```python
from build123d import *

# Parameters (mm, degrees)
F0_R     = 34.925
F0_R_2   = 16.002
F1_DEPTH = 28.829
F2_DEPTH = 7.112
F0_R_3   = 112.649
F3_DEPTH = 7.493


with BuildPart() as f1:
    # F0 (on Top) → F1 (new body, symmetric)
    with BuildSketch(Plane.XY):
        Circle(F0_R)
        Circle(F0_R_2, mode=Mode.SUBTRACT)
    extrude(amount=F1_DEPTH, both=True)

    # F0 (on Top) → F2 (join, symmetric)
    with BuildSketch(Plane.XY):
        with BuildLine():
            ThreePointArc((41.091917, -3.883291), (41.229204, -1.943802), (41.275, 0))
            ThreePointArc((41.275, 0), (33.800319, 23.688901), (14.083526, 38.797937))
            ThreePointArc((14.083526, 38.797937), (-1.674687, 41.241012), (-17.18293, 37.52829))
            ThreePointArc((-17.18293, 37.52829), (-36.553107, 19.170184), (-40.641762, -7.202277))
            ThreePointArc((-40.641762, -7.202277), (-34.87842, -22.070827), (-23.908987, -33.644999))
            ThreePointArc((-23.908987, -33.644999), (1.674687, -41.241012), (26.558236, -31.59566))
            ThreePointArc((26.558236, -31.59566), (36.553107, -19.170184), (41.091917, -3.883291))
        make_face()
        Circle(F0_R, mode=Mode.SUBTRACT)
        with BuildLine():
            ThreePointArc((-17.18293, 37.52829), (-1.674687, 41.241012), (14.083526, 38.797937))
            Line((14.083526, 38.797937), (14.083526, 96.642205))
            ThreePointArc((14.083526, 96.642205), (-4.052266, 97.578895), (-22.047948, 95.141734))
            Line((-22.047948, 95.141734), (-17.18293, 37.52829))
        make_face()
        with BuildLine():
            ThreePointArc((-23.908987, -33.644999), (-34.87842, -22.070827), (-40.641762, -7.202277))
            Line((-40.641762, -7.202277), (-90.736368, -36.124411))
            ThreePointArc((-90.736368, -36.124411), (-82.479669, -52.298813), (-71.371184, -66.66495))
            Line((-71.371184, -66.66495), (-23.908987, -33.644999))
        make_face()
        with BuildLine():
            Line((93.419133, -28.476784), (41.091917, -3.883291))
            ThreePointArc((41.091917, -3.883291), (36.553107, -19.170184), (26.558236, -31.59566))
            Line((26.558236, -31.59566), (76.652842, -60.517794))
            ThreePointArc((76.652842, -60.517794), (86.531935, -45.280082), (93.419133, -28.476784))
        make_face()
    extrude(amount=F2_DEPTH, both=True)

    # F0 (on Top) → F3 (join, symmetric)
    with BuildSketch(Plane.XY):
        Circle(F0_R_3)
        with BuildLine():
            ThreePointArc((-22.047948, 95.141734), (-4.052266, 97.578895), (14.083526, 96.642205))
            ThreePointArc((14.083526, 96.642205), (73.869821, 63.88514), (97.663, 0))
            ThreePointArc((97.663, 0), (96.596207, -14.395638), (93.419133, -28.476784))
            ThreePointArc((93.419133, -28.476784), (86.531935, -45.280082), (76.652842, -60.517794))
            ThreePointArc((76.652842, -60.517794), (4.052266, -97.578895), (-71.371184, -66.66495))
            ThreePointArc((-71.371184, -66.66495), (-82.479669, -52.298813), (-90.736368, -36.124411))
            ThreePointArc((-90.736368, -36.124411), (-86.531935, 45.280082), (-22.047948, 95.141734))
        make_face(mode=Mode.SUBTRACT)
    extrude(amount=F3_DEPTH, both=True)


solid = f1.part
```
Verification items for the finished model (mm, model axes). A direction names the side the tool comes from. Give positions to 0.01 mm unless a question says otherwise; leave off trailing zeros. Order: outer loops, then holes, each group sorted by start corner. A loop starts at its lowest first (then second) coordinate and runs counter-clockwise, first axis right, second up. Notation, with made-up numbers: (-26, 32) -> (-1, 32) arc R23 ccw to (-1, 60) -> close; hole circle Ø11 at (29.5, 86.5). An arc over 180 degrees is marked (long way). Use a Markdown table: item, result.
1) Material ranges on probe 1 along Y at (x, z) = (0, -15) (3 decimals); probe 2 along Y at (x, z) = (-34.5, 0.5); probe 3 along X at (y, z) = (0.5, 9), recorded low to high.
Results:
| item | result |
|---|---|
| probe 1 | -34.925 to -16.002, 16.002 to 34.925 |
| probe 2 | -107.24 to -91.37, -41.01 to 22.66, 91.37 to 107.24 |
| probe 3 | -34.92 to -15.99, 15.99 to 34.92 |
2) Section check D-D, the plane y = 22. Record the boundary of the cut face in (x, z), then the cut area to 3 significant figures.
Results:
| item | result |
|---|---|
| outline | (-110.48, -7.49) -> (-95.15, -7.49) -> (-95.15, 7.49) -> (-110.48, 7.49) -> close; (-34.92, -7.11) -> (-27.12, -7.11) -> (-27.12, -28.83) -> (27.12, -28.83) -> (27.12, -7.11) -> (34.92, -7.11) -> (34.92, 7.11) -> (27.12, 7.11) -> (27.12, 28.83) -> (-27.12, 28.83) -> (-27.12, 7.11) -> (-34.92, 7.11) -> close; (95.15, -7.49) -> (110.48, -7.49) -> (110.48, 7.49) -> (95.15, 7.49) -> close |
| area | 3,810 mm² |
3) Depth check by flat-ended pin: pin 1 Ø6 at (y, z) = (17, -16.5) entering from -X; pin 2 Ø1.5 at (x, y) = (71, -55) entering from +Z; pin 3 Ø1 at (y, z) = (30, -16.5) entering from +X. Enter the tip coordinate at first touch or a pass-through.
Results:
| item | result |
|---|---|
| pin 1 | x = -32 |
| pin 2 | z = 7.11 |
| pin 3 | x = 18.7 |
4) Mould release check, pull along Y, two halves, no side actions. Record for faces 5 (the cylindrical face through (-82.343, -52.514, 7.305)), 6 (the flat face through (7, -15, -28.829)): pulls with the +Y half, pulls with the -Y half, needs draft (parallel to the pull), parting line crosses it, or undercut.
Results:
| item | result |
|---|---|
| face 5 | undercut |
| face 6 | needs draft |
5) Tool access check on faces 1 (the flat face through (7, -15, 28.829)), 2 (the cylindrical face through (-27.715, -21.251, -17.818)), 3 (the flat face through (67.62, -16.35, 0.1)), 4 (the flat face through (15, -33, 7.112)). Record the directions out of +Z, -Z, +X, -X, +Y, -Y that give a thin tool (end or side, any length) a straight path to the whole face; none if there is none.
Results:
| item | result |
|---|---|
| face 1 | +Z, +X, -X, +Y, -Y |
| face 2 | -Z |
| face 3 | +Z, -Z |
| face 4 | +Z |
6) Section check A-A, the plane x = 0. Record the boundary of the cut face in (y, z) (3 decimals), then the cut area to 3 significant figures.
Results:
| item | result |
|---|---|
| outline | (-112.649, -7.493) -> (-97.663, -7.493) -> (-97.663, 7.493) -> (-112.649, 7.493) -> close; (-41.275, -7.112) -> (-34.925, -7.112) -> (-34.925, -28.829) -> (-16.002, -28.829) -> (-16.002, 28.829) -> (-34.925, 28.829) -> (-34.925, 7.112) -> (-41.275, 7.112) -> close; (16.002, -28.829) -> (34.925, -28.829) -> (34.925, -7.112) -> (97.663, -7.112) -> (97.663, -7.493) -> (112.649, -7.493) -> (112.649, 7.493) -> (97.663, 7.493) -> (97.663, 7.112) -> (34.925, 7.112) -> (34.925, 28.829) -> (16.002, 28.829) -> close |
| area | 3,610 mm² |
7) Section check C-C, the plane y = -11. Record the boundary of the cut face in (x, z).
Results:
| item | result |
|---|---|
| outline | (-112.11, -7.49) -> (-97.04, -7.49) -> (-97.04, 7.49) -> (-112.11, 7.49) -> close; (-47.22, -7.11) -> (-33.15, -7.11) -> (-33.15, -28.83) -> (-11.62, -28.83) -> (-11.62, 28.83) -> (-33.15, 28.83) -> (-33.15, 7.11) -> (-47.22, 7.11) -> close; (11.62, -28.83) -> (33.15, -28.83) -> (33.15, -7.11) -> (56.23, -7.11) -> (56.23, 7.11) -> (33.15, 7.11) -> (33.15, 28.83) -> (11.62, 28.83) -> close; (97.04, -7.49) -> (112.11, -7.49) -> (112.11, 7.49) -> (97.04, 7.49) -> close |
8) Section check B-B, the plane z = -3.5. Record the boundary of the cut face in (x, y) (3 decimals), then the cut area to 3 significant figures.
Results:
| item | result |
|---|---|
| outline | circle Ø225.298 at (0, 0); hole (-90.736, -36.124) -> (-40.642, -7.202) arc R41.275 cw to (-17.183, 37.528) -> (-22.048, 95.142) arc R97.663 ccw to start; hole (-71.371, -66.665) arc R97.663 ccw to (76.653, -60.518) -> (26.558, -31.596) arc R41.275 cw to (-23.909, -33.645) -> close; hole circle Ø32.004 at (0, 0); hole (14.084, 38.798) arc R41.275 cw to (41.275, 0) arc R41.275 cw to (41.092, -3.883) -> (93.419, -28.477) arc R97.663 ccw to (97.663, 0) arc R97.663 ccw to (14.084, 96.642) -> close |
| area | 20,200 mm² |
